Part print with two shaded views. Sizes in mm from the minimum x, y, z corner. A direction names the side the tool comes from. Coordinates: 2 decimals unless noted, no trailing zeros. Order: outer loops, then holes, each group sorted by start corner. A loop starts at its lowest first (then second) coordinate and runs counter-clockwise, first axis right, second up. Notation, with made-up numbers: (23.25, -35.5) - (56.25, -35.5) arc R20 ccw to (56.25, -21.5) - close; hole circle Ø7 at (27.25, -1). An arc over 180 degrees is marked (long way). One line per item, written item: value.
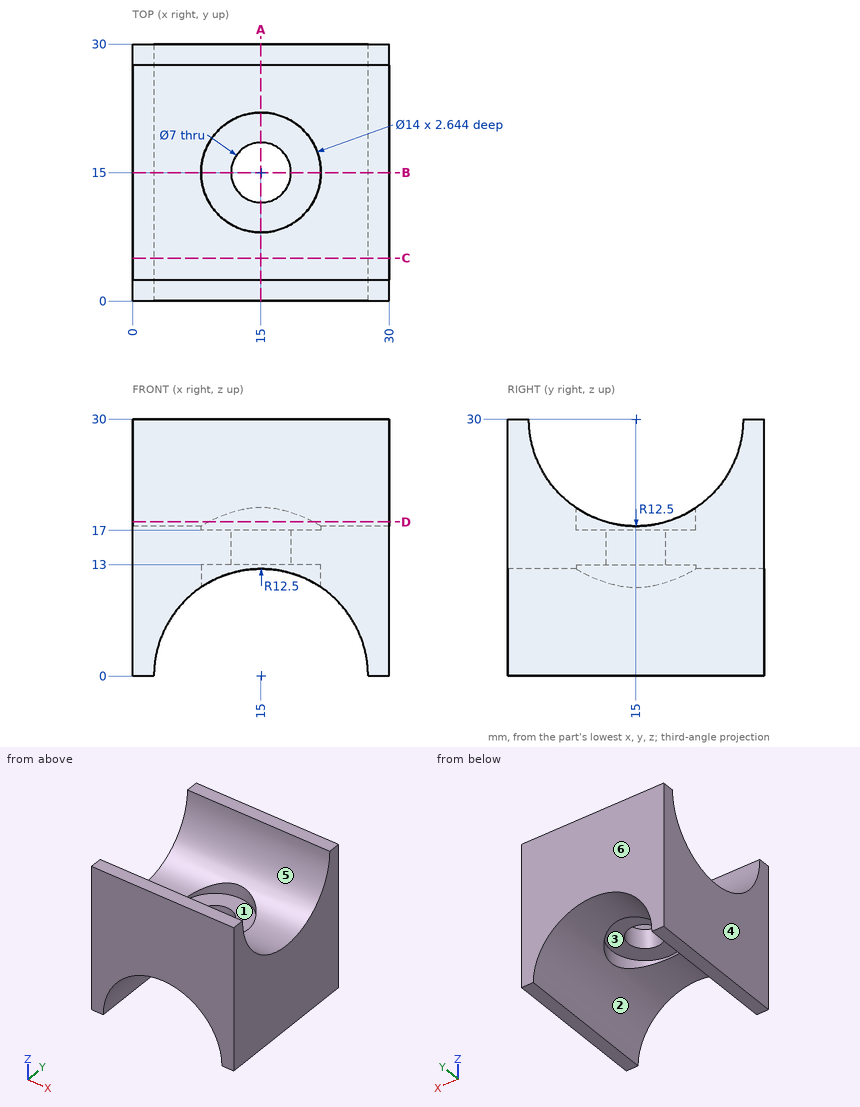
1. Flat gauge pins, fed straight in: P1, Ø7, axis at x = 17.5, y = 16.5, coming from the +Z side; P2, Ø3, axis at x = 22, y = 11, coming from the -Z side (1 decimal); P3, Ø8.5, axis at x = 15, y = 15, coming from the -Z side. Where does each tip first touch, or does it go through?
Values found:
P1: stops at z = 17
P2: stops at z = 9.2
P3: stops at z = 13
2. Two-plate mould, pull along Y, no slides. Class the marked faces 3, 4, 5 and 6: pulls with the +Y half, pulls with the -Y half, needs draft (parallel to the pull), parting line crosses it, or undercut.
Values found:
face 3: undercut
face 4: needs draft
face 5: undercut
face 6: pulls with the +Y half
3. Probe line 1 along Y through (x, z) = (15, 18); line 2 along Y through (x, z) = (15, 15.75); line 3 along Z through (x, y) = (16.5, 11.5). List the from-to ranges inside material, lowest first.
Values found:
line 1: y = 0 to 8, 22 to 30
line 2: y = 0 to 11.5, 18.5 to 30
line 3: z = 13 to 17
4. Band-saw the part on C-C, the plane y = 5. Give the cut face in (x, z).
Values found:
outline: (0, 0) - (2.5, 0) arc R12.5 cw to (27.5, 0) - (30, 0) - (30, 22.5) - (0, 22.5) - close
5. 3-axis set-ups, long thin cutter, end or side, ignore diameter. For the marked faces 1 and 2: which of +Z, -Z, +X, -X, +Y, -Y reach the whole face in a straight line?
Values found:
face 1: +Z
face 2: -Z, +Y, -Y
6. Band-saw the part on D-D, the plane z = 18. Give the cut face in (x, y).
Values found:
outline: (0, 0) - (30, 0) - (30, 11.5) - (21.06, 11.5) arc R7 cw to (8.94, 11.5) - (0, 11.5) - close; (0, 18.5) - (8.94, 18.5) arc R7 cw to (21.06, 18.5) - (30, 18.5) - (30, 30) - (0, 30) - close
7. Band-saw the part on B-B, the plane y = 15. Give the cut face in (x, z).
Values found:
outline: (0, 0) - (2.5, 0) arc R12.5 cw to (8, 10.36) - (8, 13) - (11.5, 13) - (11.5, 17) - (8, 17) - (8, 17.5) - (0, 17.5) - close; (18.5, 13) - (22, 13) - (22, 10.36) arc R12.5 cw to (27.5, 0) - (30, 0) - (30, 17.5) - (22, 17.5) - (22, 17) - (18.5, 17) - close
8. Band-saw the part on A-A, the plane x = 15. Give the cut face in (y, z).
Values found:
outline: (0, 12.5) - (8, 12.5) - (8, 13) - (11.5, 13) - (11.5, 17) - (8, 17) - (8, 19.64) arc R12.5 cw to (2.5, 30) - (0, 30) - close; (18.5, 13) - (22, 13) - (22, 12.5) - (30, 12.5) - (30, 30) - (27.5, 30) arc R12.5 cw to (22, 19.64) - (22, 17) - (18.5, 17) - close
